Design review of the part built by this model. Coordinates are the model's own, in mm. Coordinates: 2 decimals unless noted, no trailing zeros. Loops run counter-clockwise (first coordinate to the right, second up) from the corner with the lowest first, then second, coordinate; pieces in that order, holes last. Notation, with made-up numbers: (43, 17) - (99, 17) arc R15 cw to (99, 22) - close; hole circle Ø3 at (27.5, 34). An arc over 180 degrees is marked (long way). Return JSON: item names as keys, results as strings. Group by question number.
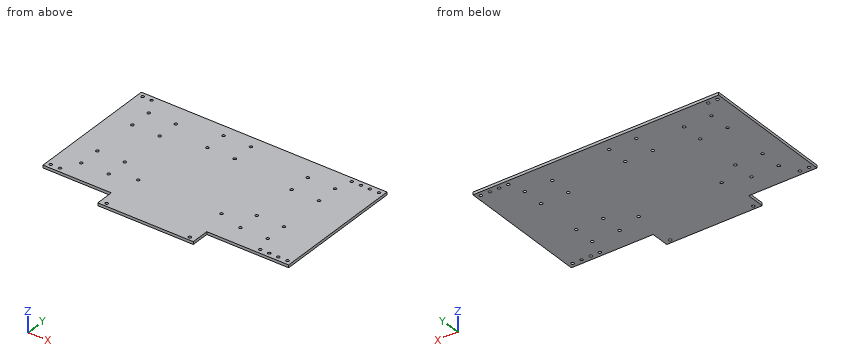
from build123d import *

# Parameters (mm, degrees)
SKETCH_1_R      = 1.6
EXTRUDE_1_DEPTH = 3


with BuildPart() as part:
    # 草图1 → 凸台-拉伸1 (new body)
    with BuildSketch(Plane.XY):
        Polygon((165.87891634, -46.129428967), (185.87891634, -46.129428967), (185.87891634, 99.870571033), (165.87891634, 99.870571033), (95.87891634, 99.870571033), (-9.12108366, 99.870571033), (-79.12108366, 99.870571033), (-84.12108366, 99.870571033), (-84.12108366, -46.129428967), (-79.12108366, -46.129428967), (-9.12108366, -46.129428967), (-9.12108366, -66.129428967), (95.87891634, -66.129428967), (95.87891634, -46.129428967), align=None)
        with Locations((-59.12108366, 0.870571033)):
            Circle(SKETCH_1_R, mode=Mode.SUBTRACT)
        with Locations((-29.12108366, 0.870571033)):
            Circle(SKETCH_1_R, mode=Mode.SUBTRACT)
        with Locations((-59.12108366, -23.129428967)):
            Circle(SKETCH_1_R, mode=Mode.SUBTRACT)
        with Locations((-29.12108366, -23.129428967)):
            Circle(SKETCH_1_R, mode=Mode.SUBTRACT)
        with Locations((115.87891634, 0.870571033)):
            Circle(SKETCH_1_R, mode=Mode.SUBTRACT)
        with Locations((145.87891634, 0.870571033)):
            Circle(SKETCH_1_R, mode=Mode.SUBTRACT)
        with Locations((115.87891634, -23.129428967)):
            Circle(SKETCH_1_R, mode=Mode.SUBTRACT)
        with Locations((145.87891634, -23.129428967)):
            Circle(SKETCH_1_R, mode=Mode.SUBTRACT)
        with Locations((-2.32108366, -62.129428967)):
            Circle(SKETCH_1_R, mode=Mode.SUBTRACT)
        with Locations((-2.32108366, -15.129428967)):
            Circle(SKETCH_1_R, mode=Mode.SUBTRACT)
        with Locations((89.07891634, -15.129428967)):
            Circle(SKETCH_1_R, mode=Mode.SUBTRACT)
        with Locations((89.07891634, -62.129428967)):
            Circle(SKETCH_1_R, mode=Mode.SUBTRACT)
        with Locations((145.87891634, 76.870571033)):
            Circle(SKETCH_1_R, mode=Mode.SUBTRACT)
        with Locations((115.87891634, 76.870571033)):
            Circle(SKETCH_1_R, mode=Mode.SUBTRACT)
        with Locations((145.87891634, 52.870571033)):
            Circle(SKETCH_1_R, mode=Mode.SUBTRACT)
        with Locations((115.87891634, 52.870571033)):
            Circle(SKETCH_1_R, mode=Mode.SUBTRACT)
        with Locations((-29.12108366, 76.870571033)):
            Circle(SKETCH_1_R, mode=Mode.SUBTRACT)
        with Locations((-59.12108366, 76.870571033)):
            Circle(SKETCH_1_R, mode=Mode.SUBTRACT)
        with Locations((-29.12108366, 52.870571033)):
            Circle(SKETCH_1_R, mode=Mode.SUBTRACT)
        with Locations((-59.12108366, 52.870571033)):
            Circle(SKETCH_1_R, mode=Mode.SUBTRACT)
        with Locations((15.87891634, 86.870571033)):
            Circle(SKETCH_1_R, mode=Mode.SUBTRACT)
        with Locations((45.87891634, 86.870571033)):
            Circle(SKETCH_1_R, mode=Mode.SUBTRACT)
        with Locations((15.87891634, 62.870571033)):
            Circle(SKETCH_1_R, mode=Mode.SUBTRACT)
        with Locations((45.87891634, 62.870571033)):
            Circle(SKETCH_1_R, mode=Mode.SUBTRACT)
        with Locations((-79.12108366, -41.129428967)):
            Circle(SKETCH_1_R, mode=Mode.SUBTRACT)
        with Locations((-69.12108366, -41.129428967)):
            Circle(SKETCH_1_R, mode=Mode.SUBTRACT)
        with Locations((-79.12108366, 94.870571033)):
            Circle(SKETCH_1_R, mode=Mode.SUBTRACT)
        with Locations((-69.12108366, 94.870571033)):
            Circle(SKETCH_1_R, mode=Mode.SUBTRACT)
        with Locations((180.87891634, -41.129428967)):
            Circle(SKETCH_1_R, mode=Mode.SUBTRACT)
        with Locations((170.87891634, -41.129428967)):
            Circle(SKETCH_1_R, mode=Mode.SUBTRACT)
        with Locations((160.87891634, -41.129428967)):
            Circle(SKETCH_1_R, mode=Mode.SUBTRACT)
        with Locations((150.87891634, -41.129428967)):
            Circle(SKETCH_1_R, mode=Mode.SUBTRACT)
        with Locations((180.87891634, 94.870571033)):
            Circle(SKETCH_1_R, mode=Mode.SUBTRACT)
        with Locations((170.87891634, 94.870571033)):
            Circle(SKETCH_1_R, mode=Mode.SUBTRACT)
        with Locations((160.87891634, 94.870571033)):
            Circle(SKETCH_1_R, mode=Mode.SUBTRACT)
        with Locations((150.87891634, 94.870571033)):
            Circle(SKETCH_1_R, mode=Mode.SUBTRACT)
    extrude(amount=EXTRUDE_1_DEPTH)


solid = part.part
Item 1: To check wall thickness, follow line 1 (X direction, y = 1, z = 2.8); line 2 (Y direction, x = -58.5, z = 0.35); line 3 (X direction, y = 86, z = 0.55). State the ranges of each line that lie inside material, in increasing order. Write a range as from..to.
Item 2: Add section A-A (x = 128). State the section outline as (y, z) points, then the cut area to 3 significant figures.
Item 3: Add section B-B (z = 1.7). Give the number of separate pieces and of enclosed holes in the cut face, then the cut area to 3 significant figures.
Item 4: For P1, Ø1.9, axis at x = 115.88, y = -23.13, coming from the +Z side; P2, Ø0.9, axis at y = -61, z = 2, coming from the +X side; P3, Ø1.5, axis at x = 124, z = 2, coming from the -Y side, all flat-tipped, find the tip position at first contact; note any pin that passes through.
Answers below:
{
 "1": {"line 1": "x = -84.12..-60.72, -57.53..-30.72, -27.53..114.28, 117.47..144.28, 147.47..185.88", "line 2": "y = -46.13..-24.6, -21.65..-0.6, 2.35..51.4, 54.35..75.4, 78.35..99.87", "line 3": "x = -84.12..14.54, 17.22..44.54, 47.22..185.88"},
 "2": {"outline": "(-46.13, 0) - (99.87, 0) - (99.87, 3) - (-46.13, 3) - close", "area": "438 mm^2"},
 "3": {"separate pieces": "1", "enclosed holes": "36", "area": "41,200 mm^2"},
 "4": {"P1": "passes through", "P2": "stops at x = 95.88", "P3": "stops at y = -46.13"}
}
